Build history of the part. All positions in model axes, mm. A direction names the side the tool comes from. Give positions to 0.01 mm unless a question says otherwise; leave off trailing zeros. One line per question, with ' | ' between items. Start each with the question number.
(1) Pin check, flat tips, straight feed: pin 1 Ø1.9 at (x, z) = (1, -87.5) entering from +Y; pin 2 Ø1.2 at (y, z) = (-1.5, -89.5) entering from -X; pin 3 Ø0.7 at (y, z) = (-1, -45.5) entering from +X. Stop position of each tip, or through.
(2) Which spindle directions (+Z, -Z, +X, -X, +Y, -Y) get a long thin tool onto all of the face, cutting with end or side? Do faces 1 (the face through (-5.51, -4.45, -66.55)), 2 (the face through (2, -4, -67)), 3 (the face through (-4, 2, -67)), 4 (the face through (4, 2, -67)). Say none if no direction does.
(3) Drill centre lines: L1, parallel to Y at x = 0, z = -32; L2, parallel to X at y = -4.25, z = -109; L3, parallel to Y at x = -5.5, z = -13. Where is each one in solid material? Low to high. Write a range as from..to.
(4) Pull direction X, two halves, no side cores. Call faces 5 (the face through (4, -2, -67)), 6 (the face through (-4, -2, -67)), 7 (the face through (-2, 4, -67)), 8 (the face through (-2, -4, -67)): +X half, -X half, draft (parallel to the pull), parting line (faces both ways), or undercut.
from build123d import *

# Parameters (mm, degrees)
BOSS_EXTRUDE1_DEPTH = 135
SKETCH2_W           = 135
SKETCH2_H           = 2.1


with BuildPart() as part:
    # Sketch1 → Boss-Extrude1 (new body)
    with BuildSketch(Plane.XY):
        with BuildLine():
            Line((-10, -3), (-10, -9))
            ThreePointArc((-10, -9), (-9.707106781, -9.707106781), (-9, -10))
            Line((-9, -10), (-3, -10))
            Line((-3, -10), (-3, -8))
            Line((-3, -8), (-6, -8))
            Line((-6, -8), (-6, -7.060660172))
            Line((-6, -7.060660172), (-2.939339828, -4))
            Line((-2.939339828, -4), (-0.519615242, -4))
            Line((-0.519615242, -4), (0, -3.7))
            Line((0, -3.7), (0.519615242, -4))
            Line((0.519615242, -4), (2.939339828, -4))
            Line((2.939339828, -4), (6, -7.060660172))
            Line((6, -7.060660172), (6, -8))
            Line((6, -8), (3, -8))
            Line((3, -8), (3, -10))
            Line((3, -10), (9, -10))
            ThreePointArc((9, -10), (9.707106781, -9.707106781), (10, -9))
            Line((10, -9), (10, -3))
            Line((10, -3), (8, -3))
            Line((8, -3), (8, -6))
            Line((8, -6), (7.060660172, -6))
            Line((7.060660172, -6), (4, -2.939339828))
            Line((4, -2.939339828), (4, -0.519615242))
            Line((4, -0.519615242), (3.7, 0))
            Line((3.7, 0), (4, 0.519615242))
            Line((4, 0.519615242), (4, 2.939339828))
            Line((4, 2.939339828), (7.060660172, 6))
            Line((7.060660172, 6), (8, 6))
            Line((8, 6), (8, 3))
            Line((8, 3), (10, 3))
            Line((10, 3), (10, 9))
            ThreePointArc((10, 9), (9.707106781, 9.707106781), (9, 10))
            Line((9, 10), (3, 10))
            Line((3, 10), (3, 8))
            Line((3, 8), (6, 8))
            Line((6, 8), (6, 7.060660172))
            Line((6, 7.060660172), (2.939339828, 4))
            Line((2.939339828, 4), (0.519615242, 4))
            Line((0.519615242, 4), (0, 3.7))
            Line((0, 3.7), (-0.519615242, 4))
            Line((-0.519615242, 4), (-2.939339828, 4))
            Line((-2.939339828, 4), (-6, 7.060660172))
            Line((-6, 7.060660172), (-6, 8))
            Line((-6, 8), (-3, 8))
            Line((-3, 8), (-3, 10))
            Line((-3, 10), (-9, 10))
            ThreePointArc((-9, 10), (-9.707106781, 9.707106781), (-10, 9))
            Line((-10, 9), (-10, 3))
            Line((-10, 3), (-8, 3))
            Line((-8, 3), (-8, 6))
            Line((-8, 6), (-7.060660172, 6))
            Line((-7.060660172, 6), (-4, 2.939339828))
            Line((-4, 2.939339828), (-4, 0.519615242))
            Line((-4, 0.519615242), (-3.7, 0))
            Line((-3.7, 0), (-4, -0.519615242))
            Line((-4, -0.519615242), (-4, -2.939339828))
            Line((-4, -2.939339828), (-7.060660172, -6))
            Line((-7.060660172, -6), (-8, -6))
            Line((-8, -6), (-8, -3))
            Line((-8, -3), (-10, -3))
        make_face()
    extrude(amount=-BOSS_EXTRUDE1_DEPTH)

    # Sketch2 → Cut-Revolve1 (revolve, cut)
    with BuildSketch(Plane(origin=(0, 0, 0), x_dir=(0, 0, -1), z_dir=(1, 0, 0)), mode=Mode.PRIVATE) as cut_revolve1_sk:
        with Locations((67.5, 1.05)):
            Rectangle(SKETCH2_W, SKETCH2_H)
    revolve(cut_revolve1_sk.sketch.rotate(Axis((0, 0, -135), (0, 0, 1)), 270), axis=Axis((0, 0, -135), (0, 0, 1)), mode=Mode.SUBTRACT)


solid = part.part
Result set:
1) pin 1: stops at y = 4 | pin 2: stops at x = -4 | pin 3: stops at x = 4
2) face 1: +Z, -Z | face 2: +Z, -Z, -Y | face 3: +Z, -Z, -X | face 4: +Z, -Z, +X
3) L1: y = -3.7..-2.1, 2.1..3.7 | L2: x = -10..-8, -5.31..-3.19, 3.19..5.31, 8..10 | L3: y = -10..-8, -6.56..-4.44, 4.44..6.56, 8..10
4) face 5: +X half | face 6: -X half | face 7: undercut | face 8: undercut
